Here's the drawing with two shaded views (mm, measured from the low corner). I have some questions. A direction names the side the tool comes from. Coordinates: 2 decimals unless noted, no trailing zeros. Order: outer loops, then holes, each group sorted by start corner. A loop starts at its lowest first (then second) coordinate and runs counter-clockwise, first axis right, second up. Notation, with made-up numbers: (53.25, 51.25) -> (104.25, 51.25) arc R18 cw to (104.25, 86.25) -> close; hole circle Ø3 at (35.25, 2). An arc over 180 degrees is marked (long way). Answer as a JSON object with one key per item and string values. Group by question number.
(1) I want a section at C-C, the plane y = 31.75. List the corners of the cut face in (x, z) for me.
(2) I want a section at A-A, the plane z = 63.5. State how many separate pieces and enclosed holes the cut face has.
(3) I need wall thicknesses on line 1 (Z direction, x = 38, y = 75); line 2 (X direction, y = 31, z = 40); line 3 (Z direction, x = 57.15, y = 74.6). Which ranges of each line are inside material? Lowest first, please.
(4) Which directions (+Z, -Z, +X, -X, +Y, -Y) give clear straight access to the entire face, cutting with the end or side of a thin tool? Please do the marked faces 1 and 2.
(5) For pin 1 (5 mm diameter, centred on x = 45.5, z = 70.5, fed in from -Y), with a flat end and sliding along its axis, tell me the tip position at first contact or that it passes through.
(6) I want a section at B-B, the plane x = 38.1. List the corners of the cut face in (y, z) for me, plus the area to 3 significant figures.
(7) If we mould it in two halves opening along X, with no side actions, what happens to the marked faces 3, 4 and 5? For each: pulls with the +X half, pulls with the -X half, needs draft (parallel to the pull), parting line crosses it, or undercut.
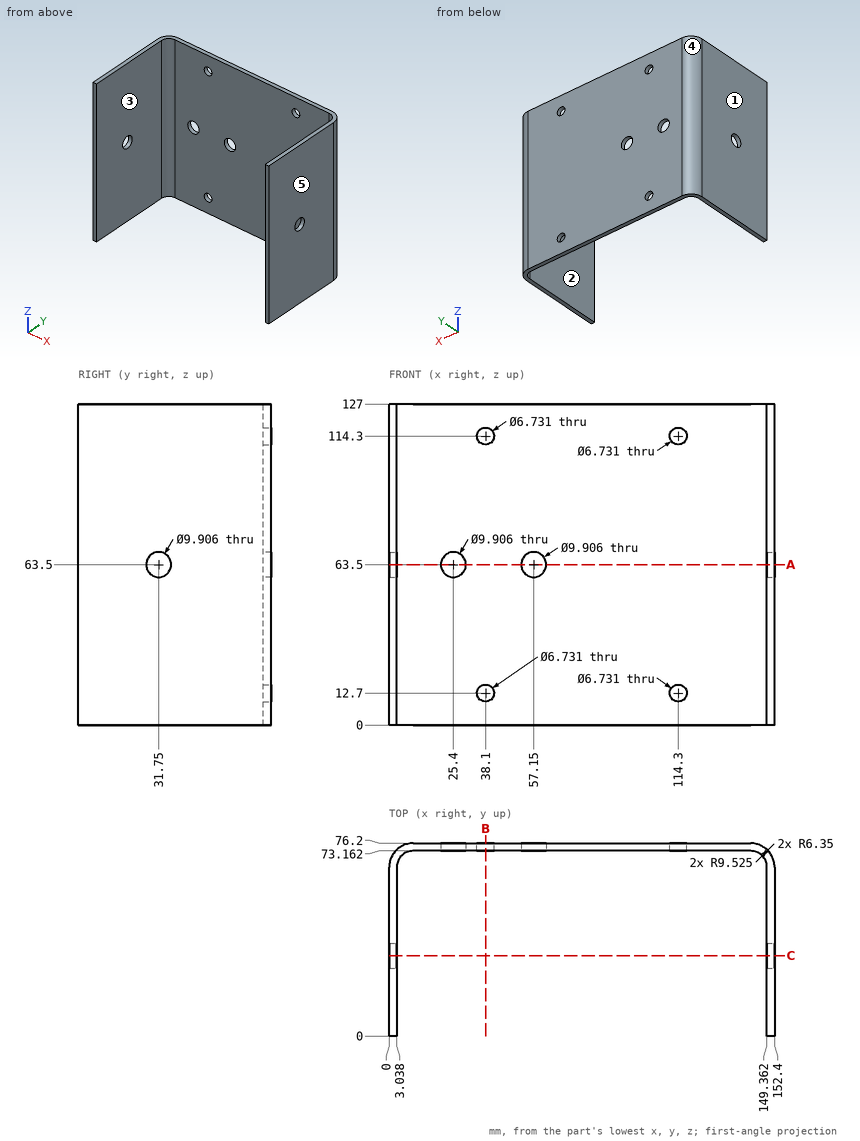
Computed values:
{
 "1": {"outline": "(0, 0) -> (3.04, 0) -> (3.04, 58.55) -> (0, 58.55) -> close; (0, 68.45) -> (3.04, 68.45) -> (3.04, 127) -> (0, 127) -> close; (149.36, 0) -> (152.4, 0) -> (152.4, 58.55) -> (149.36, 58.55) -> close; (149.36, 68.45) -> (152.4, 68.45) -> (152.4, 127) -> (149.36, 127) -> close"},
 "2": {"separate pieces": "5", "enclosed holes": "0"},
 "3": {"line 1": "z = 0 to 9.34, 16.06 to 110.94, 117.66 to 127", "line 2": "x = 0 to 3.04, 149.36 to 152.4", "line 3": "z = 0 to 58.55, 68.45 to 127"},
 "4": {"face 1": "+Z, -Z, -X, +Y, -Y", "face 2": "+Z, -Z, -Y"},
 "5": {"pin 1": "stops at y = 73.16"},
 "6": {"outline": "(73.16, 0) -> (76.2, 0) -> (76.2, 9.33) -> (73.16, 9.33) -> close; (73.16, 16.07) -> (76.2, 16.07) -> (76.2, 110.93) -> (73.16, 110.93) -> close; (73.16, 117.67) -> (76.2, 117.67) -> (76.2, 127) -> (73.16, 127) -> close", "area": "345 mm2"},
 "7": {"face 3": "undercut", "face 4": "pulls with the -X half", "face 5": "pulls with the +X half"}
}
